Answer from the drawing. Dimensions are ordinates in mm from the lowest x, y and z of the part. A direction names the side the tool comes from. Coordinates: 2 decimals unless noted, no trailing zeros. Order: outer loops, then holes, each group sorted by start corner. A loop starts at its lowest first (then second) coordinate and runs counter-clockwise, first axis right, second up. Notation, with made-up numbers: (4, 23) -> (18, 23) arc R20 ccw to (18, 48) -> close; hole circle Ø11 at (-12, 86.25). An arc over 180 degrees is marked (long way). Answer in a Markdown table with one row per item.
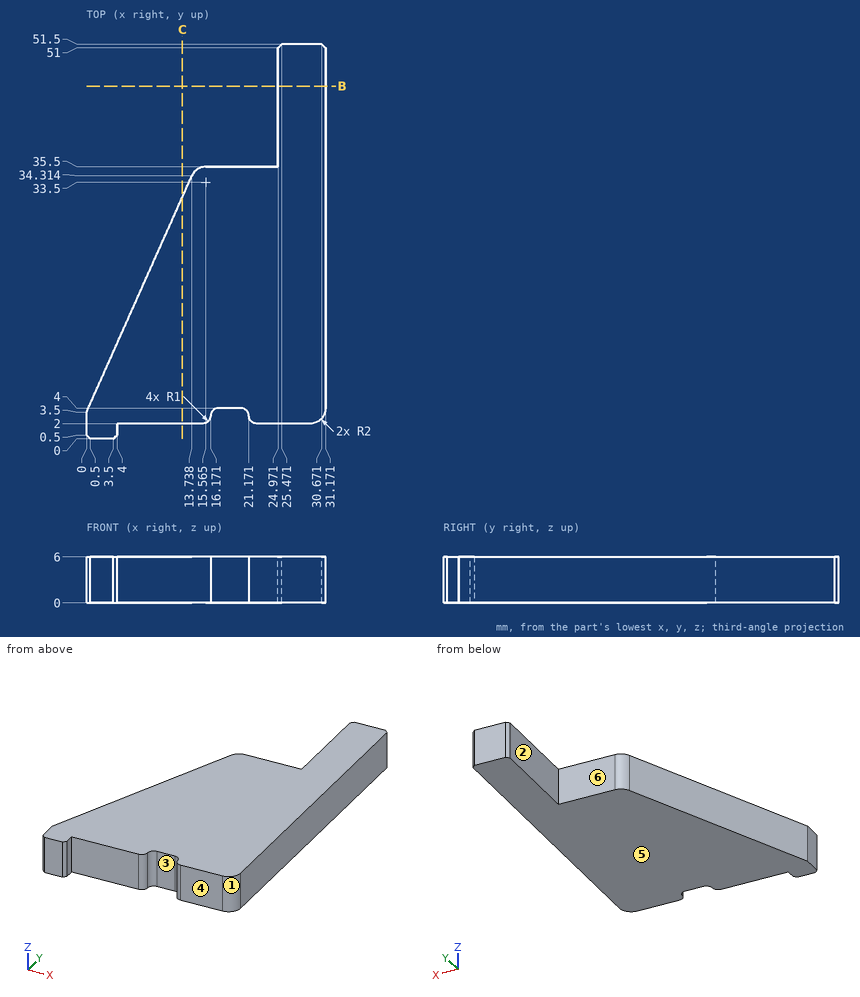
(1) A cutting plane is placed at C-C, the plane x = 12.5. Determine the outline of the cut face in (y, z).
Check values:
| item | result |
|---|---|
| outline | (2, 0) -> (31.54, 0) -> (31.54, 6) -> (2, 6) -> close |
(2) For a pull along X with two mould halves and no side action, classify the marked faces 1, 2 and 3 as released by +X, released by -X, zero draft, split by the parting line, or undercut.
Check values:
| item | result |
|---|---|
| face 1 | released by +X |
| face 2 | released by -X |
| face 3 | undercut |
(3) Flat-ended cylindrical pins translate along their axes: pin 1 (3.5 mm diameter, centred on x = 19, z = 2.5, fed in from -Y) (1 decimal); pin 2 (1.5 mm diameter, centred on y = 24, z = 4, fed in from -X) (1 decimal); pin 3 (1.8 mm diameter, centred on y = 46, z = 2, fed in from -X); pin 4 (1 mm diameter, centred on x = 21.5, y = 8, fed in from -Z). Find the tip coordinate at first contact, or state that the pin passes through.
Check values:
| item | result |
|---|---|
| pin 1 | y = 3.8 |
| pin 2 | x = 8.8 |
| pin 3 | x = 24.97 |
| pin 4 | z = 0 |
(4) A cutting plane is placed at B-B, the plane y = 46. Determine the outline of the cut face in (x, z), then the cut area to 3 significant figures.
Check values:
| item | result |
|---|---|
| outline | (24.97, 0) -> (31.17, 0) -> (31.17, 6) -> (24.97, 6) -> close |
| area | 37.2 mm² |
(5) Find the intervals of material crossed by line 1 along Y through (x, z) = (19, 2.7); line 2 along X through (y, z) = (37.5, 1.95); line 3 along Y through (x, z) = (24, 5.65), in increasing order. Write a range as from..to.
Check values:
| item | result |
|---|---|
| line 1 | 4..35.5 |
| line 2 | 24.97..31.17 |
| line 3 | 2..35.5 |
(6) Which of the six approach directions +Z, -Z, +X, -X, +Y, -Y give full straight-line access (tool end or side, diameter ignored) to the marked faces 4, 5 and 6?
Check values:
| item | result |
|---|---|
| face 4 | +Z, -Z, +X, -Y |
| face 5 | -Z, +X, -X, +Y, -Y |
| face 6 | +Z, -Z, -X, +Y |
